Could you check a few things on this model? Use its own coordinates, in mm. A direction names the side the tool comes from. Give positions to 0.01 mm unless a question says otherwise; leave off trailing zeros. Loops run counter-clockwise (first coordinate to the right, second up) from the corner with the lowest first, then second, coordinate; pieces in that order, holes last. Notation, with made-up numbers: (-35, 40.5) - (19, 40.5) arc R25 ccw to (19, 76.5) - close; hole circle Ø8 at (-23, 23.5). An arc over 180 degrees is marked (long way). Write each question's results on one line, items separated by ' | '. Start each with the question number.
(1) For pin 1 (1 mm diameter, centred on y = -4, z = 5, fed in from +X); pin 2 (1.8 mm diameter, centred on x = 1, y = -3.5, fed in from +Z); pin 3 (1 mm diameter, centred on x = 4.5, y = -0.5, fed in from +Z), each with a flat end and sliding along its axis, tell me the tip position at first contact or that it passes through.
(2) Suppose I cut it at B-B (y = -2.9). Please give me the cut outline in (x, z), and give its area (3 significant figures).
(3) On a 3-axis mill with a long thin cutter (end or side, diameter ignored), from which of +Z, -Z, +X, -X, +Y, -Y can I reach the whole of each face in a straight line? I mean faces 1 (the face through (0, -3, 7.361)), 2 (the face through (-7, -1.5, -4)), 3 (the face through (6.405, -3.226, 3.629)). Say none if no direction works.
(4) Suppose I cut it at A-A (x = 0). Please give me the cut outline in (y, z).
(5) If we mould it in two halves opening along Z, with no side actions, what happens to faces 4 (the face through (6.345, -3.226, -3.732)), 5 (the face through (4.626, -1.972, 1.457)), 6 (the face through (6, -5, 2))? For each: released by +Z, released by -Z, zero draft, split by the parting line, or undercut.
(6) I need wall thicknesses on line 1 (Z direction, x = 0, y = -1.1); line 2 (Z direction, x = 0, y = -2.3); line 3 (X direction, y = -0.15, z = 0.5). Which ranges of each line are inside material? Lowest first, please.
from build123d import *

# Parameters (mm, degrees)
SKETCH_R     = 8.75
PAD_DEPTH    = 1.5
PAD001_DEPTH = 3.5
SKETCH002_R  = 4.85
POCKET_DEPTH = 7
CHAMFER_SIZE = 1


with BuildPart() as part:
    # Sketch → Pad (new body)
    with BuildSketch(Plane.XZ):
        Circle(SKETCH_R)
    extrude(amount=PAD_DEPTH)

    # Sketch001 (on Face3 of Pad) → Pad001 (join)
    with BuildSketch(Plane.XZ.offset(1.5)):
        Polygon((8.5, 0), (4.25, 7.361216), (-4.25, 7.361216), (-8.5, 0), (-4.25, -7.361216), (4.25, -7.361216), align=None)
    extrude(amount=PAD001_DEPTH)

    # Sketch002 → Pocket (cut)
    with BuildSketch(Plane.XZ):
        Circle(SKETCH002_R)
    extrude(amount=POCKET_DEPTH, mode=Mode.SUBTRACT)

    # Chamfer
    chamfer_edges = [part.edges().sort_by_distance(p)[0] for p in [
        (-4.85, -5, 0),
    ]]
    chamfer(chamfer_edges, length=CHAMFER_SIZE)


solid = part.part
Output values:
1) pin 1: x = 5.9 | pin 2: z = 7.36 | pin 3: z = 7.78
2) outline: (-8.5, 0) - (-4.25, -7.36) - (4.25, -7.36) - (8.5, 0) - (4.25, 7.36) - (-4.25, 7.36) - close; hole circle Ø9.7 at (0, 0) | area: 114 mm2
3) face 1: +Z, +X, -X, -Y | face 2: -Y | face 3: +Z, +X, -Y
4) outline: (-5, -7.36) - (-1.5, -7.36) - (-1.5, -8.75) - (0, -8.75) - (0, -4.85) - (-4, -4.85) - (-5, -5.85) - close; (-5, 5.85) - (-4, 4.85) - (0, 4.85) - (0, 8.75) - (-1.5, 8.75) - (-1.5, 7.36) - (-5, 7.36) - close
5) face 4: released by -Z | face 5: undercut | face 6: zero draft
6) line 1: -8.75 to -4.85, 4.85 to 8.75 | line 2: -7.36 to -4.85, 4.85 to 7.36 | line 3: -8.74 to -4.82, 4.82 to 8.74
